The drawing under review shows one solid part. Ordinate dimensions are in mm from its lowest x, y, z. A direction names the side the tool comes from. Round coordinates to 2 decimals unless told otherwise and drop trailing zeros. Order: outer loops, then holes, each group sorted by start corner. A loop starts at its lowest first (then second) coordinate and runs counter-clockwise, first axis right, second up. Notation, with made-up numbers: M 66,70.25 L 120,70.25 A14 ccw 120,89.25 Z; hole C -7.75,29 d8. An arc over 180 degrees is marked long. Answer as a JSON object with one key per item and string values. Group by question number.
1. To check wall thickness, follow probe 1 along Y at (x, z) = (3.25, 4.5); probe 2 along Y at (x, z) = (8.25, 2.5); probe 3 along Z at (x, y) = (7, 13.75). State the ranges of each line that lie inside material, in increasing order. Write a range as [from, to].
2. Add section D-D on y = 8.75. State the section outline as (x, z) points.
3. Add section A-A on y = 12.5. State the section outline as (x, z) points.
4. Clearance check with flat-ended pins moving along their axes: P1, Ø4.5, axis at x = 6, z = 5, coming from the +Y side; P2, Ø0.6, axis at x = 6, y = 13.5, coming from the -Z side; P3, Ø1, axis at y = 8.5, z = 5.5, coming from the -X side. State where each tip first meets the part, or that it passes through.
5. Add section B-B on x = 5.85. State the section outline as (y, z) points.
6. Machinability: for the marked faces 1, 2, 3 and 4, which of the approach directions +Z, -Z, +X, -X, +Y, -Y give a long, thin tool a straight path to every point of the face, cutting with its end or side? Answer none if there is none.
7. Mouldability with a two-part tool opening along Y and no side actions: class the marked faces 5, 6 and 7 as released by +Y, released by -Y, zero draft, split by the parting line, or undercut.
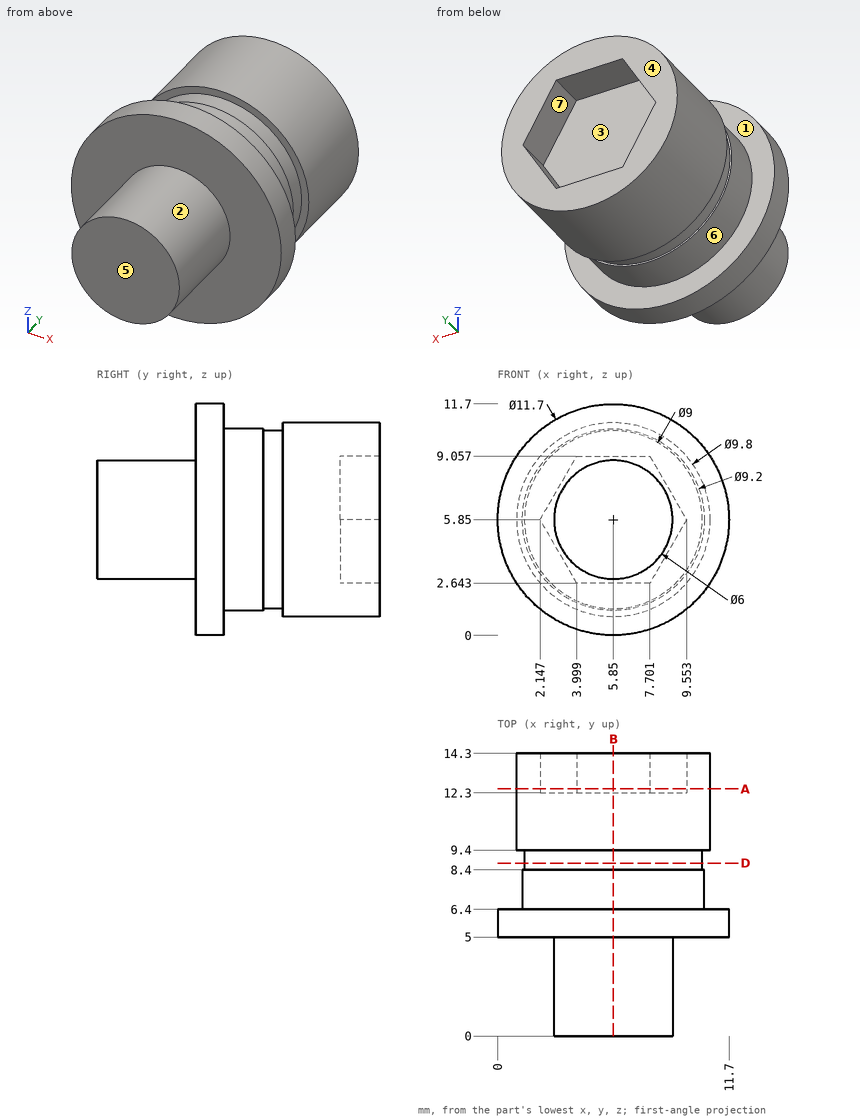
Recorded:
{
 "1": {"probe 1": "y = [0, 12.3]", "probe 2": "y = [5, 14.3]", "probe 3": "z = [1.09, 2.64], [9.06, 10.61]"},
 "2": {"outline": "C 5.85,5.85 d9"},
 "3": {"outline": "C 5.85,5.85 d9.8; hole M 2.15,5.85 L 4,2.64 L 7.7,2.64 L 9.55,5.85 L 7.7,9.06 L 4,9.06 Z"},
 "4": {"P1": "stops at y = 12.3", "P2": "stops at z = 0.95", "P3": "stops at x = 1.25"},
 "5": {"outline": "M 0,2.85 L 5,2.85 L 5,0 L 6.4,0 L 6.4,1.25 L 8.4,1.25 L 8.4,1.35 L 9.4,1.35 L 9.4,0.95 L 14.3,0.95 L 14.3,2.64 L 12.3,2.64 L 12.3,9.06 L 14.3,9.06 L 14.3,10.75 L 9.4,10.75 L 9.4,10.35 L 8.4,10.35 L 8.4,10.45 L 6.4,10.45 L 6.4,11.7 L 5,11.7 L 5,8.85 L 0,8.85 Z"},
 "6": {"face 1": "none", "face 2": "-Y", "face 3": "+Y", "face 4": "+Z, -Z, +X, -X, +Y"},
 "7": {"face 5": "released by -Y", "face 6": "undercut", "face 7": "zero draft"}
}
